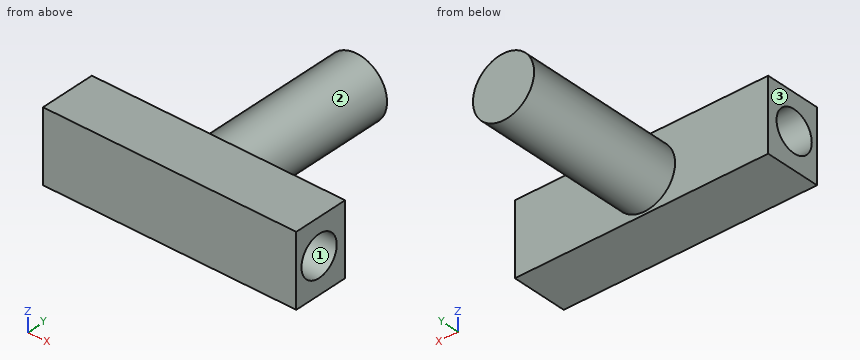
```python
from build123d import *

# Parameters (mm, degrees)
F0_W      = 119.415596
F0_H      = 33.568412
F1_DEPTH  = 1
F1_FACE_W = 119.415596
F1_FACE_H = 33.568412
F2_DEPTH  = 25.4
F4_D      = 19.05
F5_R      = 14.418988
F6_DEPTH  = 76.2


with BuildPart() as f1:
    # F0 (on Front) → F1 (new body)
    with BuildSketch(Plane.XZ):
        with Locations((1.385562, -3.563076)):
            Rectangle(F0_W, F0_H)
    extrude(amount=F1_DEPTH)

    # F1_face (on face) → F2 (join)
    with BuildSketch(Plane(origin=(1.385562, -1, -3.563076), x_dir=(1, 0, 0), z_dir=(0, -1, 0))):
        Rectangle(F1_FACE_W, F1_FACE_H)
    extrude(amount=F2_DEPTH)

    # F4 (through all)
    with Locations(Plane.YZ.offset(61.09336)):
        with Locations((-14.050731, -3.511861)):
            Hole(F4_D / 2)

    # F5 (on face) → F6 (join)
    with BuildSketch(Plane(origin=(0, 0, 0), x_dir=(-1, 0, 0), z_dir=(0, 1, 0))):
        with Locations((0, -4.649602)):
            Circle(F5_R)
    extrude(amount=F6_DEPTH)


solid = f1.part
```
Verification items for the finished model (mm, model axes). Face numbers are marked on the shaded views. Give positions to 0.01 mm unless a question says otherwise; leave off trailing zeros. Order: outer loops, then holes, each group sorted by start corner. A loop starts at its lowest first (then second) coordinate and runs counter-clockwise, first axis right, second up. Notation, with made-up numbers: (-17.5, 77) -> (-4.5, 77) arc R22 ccw to (-4.5, 86) -> close; hole circle Ø5 at (16, -29). An arc over 180 degrees is marked (long way). Use a Markdown table: item, result.
1) Material ranges on probe 1 along Y at (x, z) = (-13, -3.5); probe 2 along Y at (x, z) = (-34, -7.5); probe 3 along Y at (x, z) = (-20.5, 10), recorded low to high.
Results:
| item | result |
|---|---|
| probe 1 | -26.4 to -23.58, -4.53 to 76.2 |
| probe 2 | -26.4 to -22.7, -5.4 to 0 |
| probe 3 | -26.4 to 0 |
2) Section check D-D, the plane y = -6. Record the boundary of the cut face in (x, z), then the cut area to 3 significant figures.
Results:
| item | result |
|---|---|
| outline | (-58.32, -20.35) -> (61.09, -20.35) -> (61.09, -8.6) -> (-58.32, -8.6) -> close; (-58.32, 1.58) -> (61.09, 1.58) -> (61.09, 13.22) -> (-58.32, 13.22) -> close |
| area | 2,790 mm² |
3) Section check C-C, the plane x = 0. Record the boundary of the cut face in (y, z) (3 decimals), then the cut area to 3 significant figures.
Results:
| item | result |
|---|---|
| outline | (-26.4, -20.347) -> (0, -20.347) -> (0, -19.069) -> (76.2, -19.069) -> (76.2, 9.769) -> (0, 9.769) -> (0, 13.221) -> (-26.4, 13.221) -> close; hole circle Ø19.05 at (-14.051, -3.512) |
| area | 2,800 mm² |
4) Section check A-A, the plane z = -1. Record the boundary of the cut face in (x, y).
Results:
| item | result |
|---|---|
| outline | (-58.32, -26.4) -> (61.09, -26.4) -> (61.09, -23.24) -> (-58.32, -23.24) -> close; (-58.32, -4.86) -> (61.09, -4.86) -> (61.09, 0) -> (13.95, 0) -> (13.95, 76.2) -> (-13.95, 76.2) -> (-13.95, 0) -> (-58.32, 0) -> close |
5) Section check B-B, the plane y = -20. Record the boundary of the cut face in (x, z).
Results:
| item | result |
|---|---|
| outline | (-58.32, -20.35) -> (61.09, -20.35) -> (61.09, -10.95) -> (-58.32, -10.95) -> close; (-58.32, 3.93) -> (61.09, 3.93) -> (61.09, 13.22) -> (-58.32, 13.22) -> close |
6) Mould release check, pull along Z, two halves, no side actions. Record for the marked faces 1, 2 and 3: pulls with the +Z half, pulls with the -Z half, needs draft (parallel to the pull), parting line crosses it, or undercut.
Results:
| item | result |
|---|---|
| face 1 | undercut |
| face 2 | parting line crosses it |
| face 3 | needs draft |
7) Depth check by flat-ended pin: pin 1 Ø3 at (y, z) = (44.5, -6) entering from +X; pin 2 Ø5 at (x, y) = (-14, 4) entering from -Z; pin 3 Ø17 at (y, z) = (-14.05, -3.51) entering from -X; pin 4 Ø12 at (y, z) = (60.5, 8.5) entering from -X. Enter the tip coordinate at first touch or a pass-through.
Results:
| item | result |
|---|---|
| pin 1 | x = 14.42 |
| pin 2 | z = -13.35 |
| pin 3 | through |
| pin 4 | x = -12.52 |
